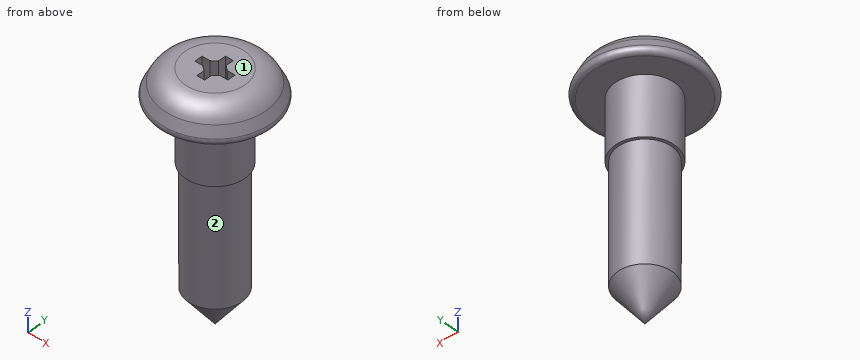
from build123d import *

# Parameters (mm, degrees)
F0_R      = 3.175
F2_R      = 2.38125
F4_R      = 1.27
F5_R      = 0.254
F7_DEPTH  = 1.5875
F8_R      = 1.5875
F9_DEPTH  = 3.175
F10_R     = 1.4422766601
F11_DEPTH = 6.35


# Not quite as in the source:
# - a length typed as a fraction of an inch, garbled in the dataset ("3 / 203.2 mm" for 3/8 in), is restored


with BuildPart() as f3:
    # F0 (on Top) → F3 section 0
    with BuildSketch(Plane.XY):
        Circle(F0_R)
    # F2 (on offset) → F3 section 1
    with BuildSketch(Plane.XY.offset(1.5875)):
        Circle(F2_R)
    loft()

    # F4
    f4_edges = [f3.edges().sort_by_distance(p)[0] for p in [
        (-2.38125, 0, 1.5875),
    ]]
    fillet(f4_edges, radius=F4_R)

    # F5
    f5_edges = [f3.edges().sort_by_distance(p)[0] for p in [
        (-3.175, 0, 0),
    ]]
    fillet(f5_edges, radius=F5_R)

    # F6 (on face) → F7 (cut)
    with BuildSketch(Plane.XY.offset(1.5875)):
        Polygon((-0.2111591544, 0.8412458697), (-0.2111591544, 0.4189275609), (-0.4643816895, 0.2111591544), (-0.8866999983, 0.2111591544), (-0.8866999983, -0.2111591544), (-0.4643816895, -0.2111591544), (-0.2111591544, -0.4189275609), (-0.2111591544, -0.8412458697), (0.2111591544, -0.8412458697), (0.2111591544, -0.4189275609), (0.4643816895, -0.2111591544), (0.8866999983, -0.2111591544), (0.8866999983, 0.2111591544), (0.4643816895, 0.2111591544), (0.2111591544, 0.4189275609), (0.2111591544, 0.8412458697), align=None)
    extrude(amount=-F7_DEPTH, mode=Mode.SUBTRACT)

    # F8 (on Top) → F9 (join)
    with BuildSketch(Plane.XY):
        Circle(F8_R)
    extrude(amount=-F9_DEPTH)

    # F10 (on face) → F11 (join)
    with BuildSketch(Plane(origin=(0, 0, -3.175), x_dir=(1, 0, 0), z_dir=(0, 0, -1))):
        Circle(F10_R)
    extrude(amount=F11_DEPTH)

    # F12 (on Right) → F13 (revolve)
    with BuildSketch(Plane.YZ):
        Polygon((0, -11.43), (1.4422766601, -9.525), (0, -9.525), align=None)
    revolve(axis=Axis((0, 0, -10.4775), (0, 0, 1)))


solid = f3.part
Input: part model. Units: mm. Frame: model coordinates. Face numbers are marked on the shaded views. A direction names the side the tool comes from. Give positions to 0.01 mm unless a question says otherwise; leave off trailing zeros. Order: outer loops, then holes, each group sorted by start corner. A loop starts at its lowest first (then second) coordinate and runs counter-clockwise, first axis right, second up. Notation, with made-up numbers: (-11.75, 72) - (-3.75, 72) arc R21 cw to (-3.75, 85) - close; hole circle Ø5 at (-27, -14.75). An arc over 180 degrees is marked (long way). Write each question's results on one line, items separated by ' | '.
Item 1: Section B-B (z = -7.25). Return loops of the section in (x, y), and give its area (3 significant figures).
A:
outline: circle Ø2.88 at (0, 0) | area: 6.54 mm^2
Item 2: Section C-C (z = -10). Return loops of the section in (x, y).
A:
outline: circle Ø2.17 at (0, 0)
Item 3: Contact query for flat-ended pins moving along their axis: pin 1 Ø0.8 at (x, y) = (0, 0) entering from +Z; pin 2 Ø0.5 at (y, z) = (-0.5, 1) entering from +X; pin 3 Ø0.5 at (y, z) = (0.5, 1) entering from -X; pin 4 Ø1.5 at (x, z) = (2.5, -1) entering from -Y. Output: stop coordinate, or through.
A:
pin 1: stops at z = 0 | pin 2: stops at x = 2.76 | pin 3: stops at x = -2.76 | pin 4: passes through
Item 4: Material intervals for line 1 along Y through (x, z) = (0, -2.5); line 2 along Y through (x, z) = (0, 0.75); line 3 along Z through (x, y) = (-1.5, -2.5), sorted ascending.
A:
line 1: y = -1.59 to 1.59 | line 2: y = -2.8 to -0.84, 0.84 to 2.8 | line 3: z = 0.05 to 0.52
Item 5: Section A-A (z = 0.5). Return loops of the section in (x, y) (3 decimals), and give its area (3 significant figures).
A:
outline: circle Ø5.85 at (0, 0); hole (-0.887, -0.211) - (-0.464, -0.211) - (-0.211, -0.419) - (-0.211, -0.841) - (0.211, -0.841) - (0.211, -0.419) - (0.464, -0.211) - (0.887, -0.211) - (0.887, 0.211) - (0.464, 0.211) - (0.211, 0.419) - (0.211, 0.841) - (-0.211, 0.841) - (-0.211, 0.419) - (-0.464, 0.211) - (-0.887, 0.211) - close | area: 25.5 mm^2
Item 6: Access query for the marked faces 1 and 2. Directions: +Z, -Z, +X, -X, +Y, -Y. A direction counts if a zero-diameter tool reaches every point of the face in a straight line with its end or side. Return the directions, or none.
A:
face 1: +Z, +X, -X, +Y, -Y | face 2: -Z
